Autodesk Inventor part; units mm, degrees
ref_plane "YZ Plane" through (0, 0, 0) normal (1, 0, 0) x (0, 1, 0)
ref_plane "XZ Plane" through (0, 0, 0) normal (0, 1, 0) x (-1, 0, 0)
ref_plane "XY Plane" through (0, 0, 0) normal (0, 0, 1) x (1, 0, 0)
sketch "Boceto1" plane through (0, 0, 0) normal (0, 0, 1) x (1, 0, 0)
  line L0 (0, 0) -> (385, 0)
  line L1 (385, 0) -> (385, 40)
  line L2 (385, 40) -> (0, 40)
  line L3 (0, 40) -> (0, 0)
  line L4 (0, 20) -> (385, 20) construction
  circle A0 centre (35, 20) radius 5
  circle A1 centre (192.5, 20) radius 5
  circle A2 centre (350, 20) radius 5
  dimension "d0" = 40
  dimension "d1" = 385
  dimension "d2" = 10
  dimension "d3" = 10
  dimension "d4" = 10
  dimension "d5" = 35
  dimension "d6" = 35
extrude "Extrusión1" add sketch "Boceto1" along normal blind 5
sketch "Boceto2" plane through (0, 0, 5) normal (0, 0, 1) x (1, 0, 0)
  circle A0 centre (65, 19) radius 3
  circle A1 centre (95, 23) radius 3
  circle A2 centre (125, 19) radius 3
  circle A3 centre (260, 19) radius 3
  circle A4 centre (290, 23) radius 3
  circle A5 centre (320, 19) radius 3
  line L0 (0, 40) -> (0, 0)
  line L1 (385, 0) -> (385, 40)
  line L2 (0, 0) -> (385, 0)
  dimension "d14" = 6
  dimension "d15" = 6
  dimension "d17" = 6
  dimension "d18" = 30
  dimension "d20" = 60
  dimension "d21" = 30
  dimension "d26" = 4
  dimension "d27" = 4
  dimension "d28" = 65
  dimension "d29" = 65
  dimension "d30" = 19
  dimension "d31" = 19
  dimension "d32" = 60
extrude "Extrusión2" cut sketch "Boceto2" against normal blind 10
properties part number "Sup.Acrilico" material "Acrílico, claro"
Here's how the part is built. I have some questions about the finished solid (model axes, mm). Round coordinates to 2 decimals unless told otherwise and drop trailing zeros. Loops run counter-clockwise (first coordinate to the right, second up) from the corner with the lowest first, then second, coordinate; pieces in that order, holes last. Notation, with made-up numbers: (6.5, 70.25) -> (12.5, 70.25) arc R20 cw to (12.5, 96.25) -> close; hole circle Ø2 at (42, 5). An arc over 180 degrees is marked (long way). Write each question's results on one line, items separated by ' | '.
(1) For P1, Ø5, axis at x = 95, y = 23, coming from the -Z side, with a flat end and sliding along its axis, tell me the tip position at first contact or that it passes through.
Worked answers:
P1: through
(2) We'd pull the mould along X, two halves only. Please class faces 1 (the face through (190, 25, 0)), 2 (the face through (92, 23, 3)): released by +X, released by -X, zero draft, split by the parting line, or undercut.
Worked answers:
face 1: zero draft | face 2: undercut
(3) If we section it at B-B, the plane z = 3.2: Give the number of separate pieces and of enclosed holes in the cut face, then the cut area to 3 significant figures.
Worked answers:
separate pieces: 1 | enclosed holes: 9 | area: 15,000 mm2
(4) If I drill on L1, parallel to Y at x = 35, z = 2.2; L2, parallel to Y at x = 65, z = 2.95; L3, parallel to X at y = 24.5, z = 0.6, over which ranges is the centre line in solid material (lowest first)?
Worked answers:
L1: 0 to 15, 25 to 40 | L2: 0 to 16, 22 to 40 | L3: 0 to 32.82, 37.18 to 92.4, 97.6 to 190.32, 194.68 to 287.4, 292.6 to 347.82, 352.18 to 385
(5) If we section it at A-A, the plane x = 350: List the corners of the cut face in (y, z) for me, then the cut area to 3 significant figures.
Worked answers:
outline: (0, 0) -> (15, 0) -> (15, 5) -> (0, 5) -> close; (25, 0) -> (40, 0) -> (40, 5) -> (25, 5) -> close | area: 150 mm2
